Can you work these out from the model? Positions are in its coordinate system, mm. Face numbers are marked on the shaded views. Coordinates: 2 decimals unless noted, no trailing zeros. Order: outer loops, then holes, each group sorted by start corner. A loop starts at its lowest first (then second) coordinate and runs counter-clockwise, first axis right, second up. Notation, with made-up numbers: (-39.75, -9) - (-27.75, -9) arc R21 cw to (-27.75, 8) - close; hole circle Ø4 at (-35, 65). An arc over 180 degrees is marked (long way). Return JSON: item names as keys, results as strings. Group by question number.
1) For pin 1 Ø8 at (x, y) = (-34.5, 90.5) entering from -Z; pin 2 Ø2 at (x, z) = (-36.5, -18) entering from +Y; pin 3 Ø2 at (x, y) = (-4.5, 141) entering from -Z, each with a flat end and sliding along its axis, tell me the tip position at first contact or that it passes through.
2) If we mould it in two halves opening along Z, with no side actions, what happens to the marked faces 1 and 2? For each: pulls with the +Z half, pulls with the -Z half, needs draft (parallel to the pull), parting line crosses it, or undercut.
3) Imagine slicing it at A-A (x = 7). Write out the boundary of the cut face in (y, z), and give its area (3 significant figures).
4) If I drill on line 1 along Z through (x, y) = (51, -8.5); line 2 along Y through (x, z) = (58, 0); line 3 along Y through (x, z) = (-74.5, -43), over which ranges is the centre line in solid material (lowest first)?
5) Imagine slicing it at B-B (x = -22.5). Write out the boundary of the cut face in (y, z).
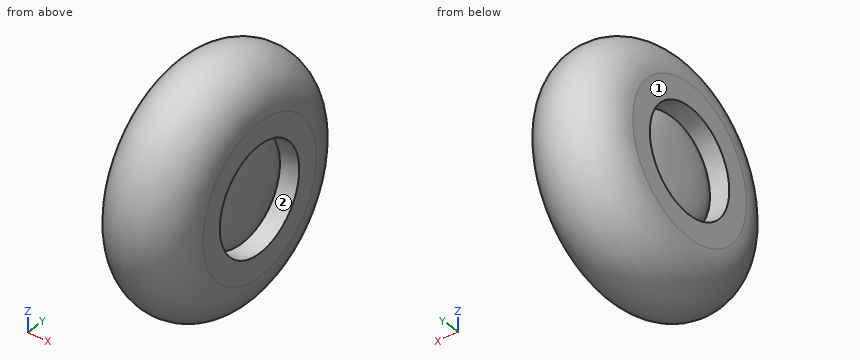
```python
from build123d import *


with BuildPart() as part:
    # Sketch3 → Revolve1 (revolve)
    with BuildSketch(Plane.XY, mode=Mode.PRIVATE) as revolve1_sk:
        with BuildLine():
            Line((-66.675, 0), (66.675, 0))
            add(Edge.make_bspline(
                [(44.45, 104.4575), (66.90298373, 104.4575), (66.675, 43.682715928), (66.675, 0)],
                knots=[0, 0, 0, 0, 1, 1, 1, 1], degree=3))
            Line((44.45, 104.4575), (88.9, 104.4575))
            Line((88.9, 104.4575), (88.9, 149.225))
            ThreePointArc((88.9, 149.225), (0, 238.125), (-88.9, 149.225))
            Line((-88.9, 149.225), (-88.9, 104.4575))
            Line((-88.9, 104.4575), (-44.45, 104.4575))
            add(Edge.make_bspline(
                [(-44.45, 104.4575), (-66.90298373, 104.4575), (-66.675, 43.682715928), (-66.675, 0)],
                knots=[0, 0, 0, 0, 1, 1, 1, 1], degree=3))
        make_face()
    revolve(revolve1_sk.sketch.rotate(Axis((0, 0, 0), (1, 0, 0)), 90), axis=Axis((0, 0, 0), (1, 0, 0)))


solid = part.part
```
Calculated:
{
 "1": {"pin 1": "z = -215.11", "pin 2": "y = 230.03", "pin 3": "z = -192.48"},
 "2": {"face 1": "needs draft", "face 2": "undercut"},
 "3": {"outline": "circle Ø475.7 at (0, 0)", "area": "178,000 mm2"},
 "4": {"line 1": "-221.88 to -104.11, -102.05 to 102.05, 104.11 to 221.88", "line 2": "-216.6 to -104.46, -92.99 to 92.99, 104.46 to 216.6", "line 3": "-193 to -95.2, 95.2 to 193"},
 "5": {"outline": "circle Ø470.46 at (0, 0)"}
}
